Read the model definition and answer for the solid it produces. Units are mm, in the model's axes. Face numbers are marked on the shaded views. A direction names the side the tool comes from. Coordinates: 2 decimals unless noted, no trailing zeros. Order: outer loops, then holes, each group sorted by start corner. A loop starts at its lowest first (then second) coordinate and runs counter-clockwise, first axis right, second up. Notation, with made-up numbers: (76.25, 16) -> (102.25, 16) arc R15 cw to (102.25, 27) -> close; hole circle Ø4 at (69.5, 59.5). An arc over 180 degrees is marked (long way). Return JSON: item names as keys, results as strings. Group by question number.
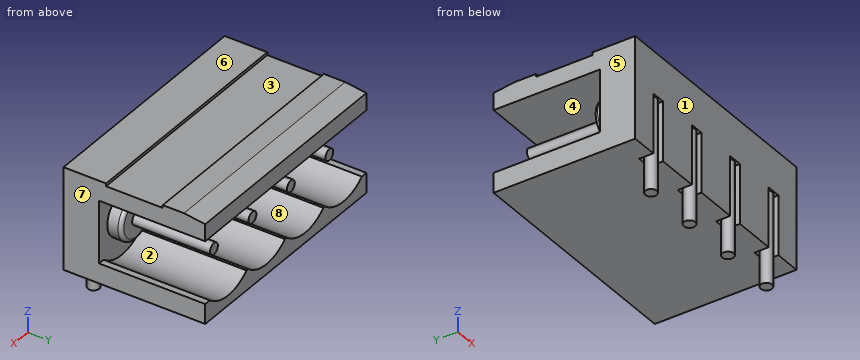
```python
from build123d import *

# Parameters (mm, degrees)
SKETCH_1_W          = 16.6
SKETCH_1_H          = 10
EXTRUDE_1_DEPTH     = 7.2
SKETCH_2_W          = 1.17709233
SKETCH_2_H          = 4
CUT_EXTRUDE_1_DEPTH = 21.673654733
CUT_EXTRUDE_2_DEPTH = 21.673654733
CUT_EXTRUDE_4_DEPTH = 7.5
SKETCH_12_R         = 0.4
EXTRUDE_8_DEPTH     = 6.5
SKETCH_13_R         = 1.5
EXTRUDE_9_DEPTH     = 1
FILLET_2_R          = 0.25
SKETCH_14_W         = 1
SKETCH_14_H         = 4.2
CUT_EXTRUDE_7_DEPTH = 1
SKETCH_15_R         = 0.4
EXTRUDE_10_DEPTH    = 6.5
CUT_EXTRUDE_9_DEPTH = 7.5


with BuildPart() as part:
    # 草图1 → 凸台-拉伸1 (new body)
    with BuildSketch(Plane.XY):
        with Locations((8.3, 5)):
            Rectangle(SKETCH_1_W, SKETCH_1_H)
    extrude(amount=EXTRUDE_1_DEPTH)

    # 草图2 → 切除-拉伸1 (cut, through all)
    with BuildSketch(Plane(origin=(16.6, 0, 0), x_dir=(0, 0, -1), z_dir=(1, 0, 0))):
        with Locations((-7.588546165, 5)):
            Rectangle(SKETCH_2_W, SKETCH_2_H)
    extrude(amount=-CUT_EXTRUDE_1_DEPTH, mode=Mode.SUBTRACT)

    # 草图3 → 切除-拉伸2 (cut, through all)
    with BuildSketch(Plane(origin=(16.6, 0, 0), x_dir=(0, 0, -1), z_dir=(1, 0, 0))):
        Polygon((-7, 10), (-7.2, 8.5), (-7.2, 10), align=None)
    extrude(amount=-CUT_EXTRUDE_2_DEPTH, mode=Mode.SUBTRACT)

    # 草图6 → 切除-拉伸4 (cut)
    with BuildSketch(Plane(origin=(0, 10, 0), x_dir=(1, 0, 0), z_dir=(0, 1, 0))):
        Polygon((0.5, -1.4), (0.391822444, -1.4), (0, -1.4), (0, -5.8), (0.391822444, -5.8), (0.5, -5.8), (16.6, -5.8), (16.6, -1.4), align=None)
    extrude(amount=-CUT_EXTRUDE_4_DEPTH, mode=Mode.SUBTRACT)

    # 草图12 → 凸台-拉伸8 (add)
    with BuildSketch(Plane(origin=(0, 2.5, 0), x_dir=(1, 0, 0), z_dir=(0, 1, 0))):
        with Locations(Location((6.32, -3.6, 0), (0, 0, 270))):
            Circle(SKETCH_12_R)
        with Locations(Location((2.36, -3.6, 0), (0, 0, 270))):
            Circle(SKETCH_12_R)
        with Locations(Location((14.24, -3.6, 0), (0, 0, 90))):
            Circle(SKETCH_12_R)
        with Locations(Location((10.28, -3.6, 0), (0, 0, 90))):
            Circle(SKETCH_12_R)
    extrude(amount=EXTRUDE_8_DEPTH)

    # 草图13 → 凸台-拉伸9 (add)
    with BuildSketch(Plane(origin=(0, 2.5, 0), x_dir=(1, 0, 0), z_dir=(0, 1, 0))):
        with Locations(Location((14.24, -3.6, 0), (0, 0, 270))):
            Circle(SKETCH_13_R)
        with Locations(Location((10.28, -3.6, 0), (0, 0, 270))):
            Circle(SKETCH_13_R)
        with Locations(Location((6.32, -3.6, 0), (0, 0, 270))):
            Circle(SKETCH_13_R)
        with Locations(Location((2.36, -3.6, 0), (0, 0, 270))):
            Circle(SKETCH_13_R)
    extrude(amount=EXTRUDE_9_DEPTH)

    # 圆角2
    fillet_2_edges = [part.edges().sort_by_distance(p)[0] for p in [
        (14.24, 3.5, 2.1),
        (10.28, 3.5, 2.1),
        (6.32, 3.5, 2.1),
        (2.36, 3.5, 2.1),
    ]]
    fillet(fillet_2_edges, radius=FILLET_2_R)

    # 草图14 → 切除-拉伸7 (cut)
    with BuildSketch(Plane.XZ):
        with Locations((2.36, 2.1)):
            Rectangle(SKETCH_14_W, SKETCH_14_H)
        with Locations((6.32, 2.1)):
            Rectangle(SKETCH_14_W, SKETCH_14_H)
        with Locations((10.28, 2.1)):
            Rectangle(SKETCH_14_W, SKETCH_14_H)
        with Locations((14.24, 2.1)):
            Rectangle(SKETCH_14_W, SKETCH_14_H)
    extrude(amount=-CUT_EXTRUDE_7_DEPTH, mode=Mode.SUBTRACT)

    # 草图15 → 凸台-拉伸10 (add)
    with BuildSketch(Plane(origin=(0, 0, 4.2), x_dir=(-1, 0, 0), z_dir=(0, 0, -1))):
        with Locations(Location((-2.36, 0.5, 0), (0, 0, 180))):
            Circle(SKETCH_15_R)
        with Locations(Location((-6.32, 0.5, 0), (0, 0, 180))):
            Circle(SKETCH_15_R)
        with Locations((-10.28, 0.5)):
            Circle(SKETCH_15_R)
        with Locations((-14.24, 0.5)):
            Circle(SKETCH_15_R)
    extrude(amount=EXTRUDE_10_DEPTH)

    # 草图16 → 切除-拉伸9 (cut)
    with BuildSketch(Plane(origin=(0, 10, 0), x_dir=(1, 0, 0), z_dir=(0, 1, 0))):
        with BuildLine():
            Line((0.470555637, -1.4), (4.249444363, -1.4))
            ThreePointArc((4.249444363, -1.4), (2.36, -0.7), (0.470555637, -1.4))
        make_face()
        with BuildLine():
            Line((12.350555637, -1.4), (16.129444363, -1.4))
            ThreePointArc((16.129444363, -1.4), (14.24, -0.7), (12.350555637, -1.4))
        make_face()
        with BuildLine():
            Line((8.390555637, -1.4), (12.169444363, -1.4))
            ThreePointArc((12.169444363, -1.4), (10.28, -0.7), (8.390555637, -1.4))
        make_face()
        with BuildLine():
            Line((4.430555637, -1.4), (8.209444363, -1.4))
            ThreePointArc((8.209444363, -1.4), (6.32, -0.7), (4.430555637, -1.4))
        make_face()
    extrude(amount=-CUT_EXTRUDE_9_DEPTH, mode=Mode.SUBTRACT)


solid = part.part
```
1. Find section D-D on y = 8.25. Determine the outline of the cut face in (x, z), and give its area (3 significant figures).
2. Find section B-B on z = -0.5. Determine the outline of the cut face in (x, y), and give its area (3 significant figures).
3. Straight lines are drawn through the part: L1, parallel to Z at x = 8.25, y = 6.5; L2, parallel to Z at x = 12.75, y = 6.25; L3, parallel to X at y = 9.75, z = 1. For each, find the intervals that lie inside material, in ascending order.
4. Which of the six approach directions +Z, -Z, +X, -X, +Y, -Y give full straight-line access (tool end or side, diameter ignored) to the marked faces 1, 2, 3 and 4?
5. Find section A-A on y = 5.25. Determine the outline of the cut face in (x, z).
6. For a pull along X with two mould halves and no side action, classify the marked faces 5, 6, 7 and 8 as released by +X, released by -X, zero draft, split by the parting line, or undercut.
7. Given pin 1 (4 mm diameter, centred on x = 5.5, y = 6.5, fed in from +Z); pin 2 (1 mm diameter, centred on y = 5.5, z = -1, fed in from -X); pin 3 (2 mm diameter, centred on x = 7.5, z = 3, fed in from +Y); pin 4 (1.5 mm diameter, centred on x = 14.5, y = 3.5, fed in from -Z), each flat-ended and moving along its own axis, determine where each tip first touches the part or whether it passes through.
Result:
{
 "1": {"outline": "(0, 0) -> (16.6, 0) -> (16.6, 1.4) -> (16.13, 1.4) arc R2.9 cw to (12.35, 1.4) -> (12.17, 1.4) arc R2.9 cw to (8.39, 1.4) -> (8.21, 1.4) arc R2.9 cw to (4.43, 1.4) -> (4.25, 1.4) arc R2.9 cw to (0.47, 1.4) -> (0, 1.4) -> close; (0, 5.8) -> (16.6, 5.8) -> (16.6, 7.2) -> (0, 7.2) -> close; circle Ø0.8 at (2.36, 3.6); circle Ø0.8 at (6.32, 3.6); circle Ø0.8 at (10.28, 3.6); circle Ø0.8 at (14.24, 3.6)", "area": "41.2 mm^2"},
 "2": {"outline": "circle Ø0.8 at (2.36, 0.5); circle Ø0.8 at (6.32, 0.5); circle Ø0.8 at (10.28, 0.5); circle Ø0.8 at (14.24, 0.5)", "area": "2.01 mm^2"},
 "3": {"L1": "0 to 1.4, 5.8 to 7", "L2": "0 to 1.11, 5.8 to 7", "L3": "0 to 1.08, 3.64 to 5.04, 7.6 to 9, 11.56 to 12.96, 15.52 to 16.6"},
 "4": {"face 1": "+Z, -Z, +X, -X, -Y", "face 2": "+Y", "face 3": "+Z, +X, -X", "face 4": "+X, -X, +Y"},
 "5": {"outline": "(0, 0) -> (16.6, 0) -> (16.6, 1.4) -> (16.13, 1.4) arc R2.9 cw to (12.35, 1.4) -> (12.17, 1.4) arc R2.9 cw to (8.39, 1.4) -> (8.21, 1.4) arc R2.9 cw to (4.43, 1.4) -> (4.25, 1.4) arc R2.9 cw to (0.47, 1.4) -> (0, 1.4) -> close; (0, 5.8) -> (16.6, 5.8) -> (16.6, 7) -> (0, 7) -> close; circle Ø0.8 at (2.36, 3.6); circle Ø0.8 at (6.32, 3.6); circle Ø0.8 at (10.28, 3.6); circle Ø0.8 at (14.24, 3.6)"},
 "6": {"face 5": "released by -X", "face 6": "zero draft", "face 7": "released by +X", "face 8": "undercut"},
 "7": {"pin 1": "z = 7.2", "pin 2": "through", "pin 3": "y = 9", "pin 4": "z = 0"}
}
